Verification items for this drawing (mm, ordinates from the low corner). Coordinates: 2 decimals unless noted, no trailing zeros. Order: outer loops, then holes, each group sorted by start corner. A loop starts at its lowest first (then second) coordinate and runs counter-clockwise, first axis right, second up. Notation, with made-up numbers: (-32.5, 6) -> (-11.5, 6) arc R14 ccw to (-11.5, 14) -> close; hole circle Ø2 at (36.25, 18). An arc over 180 degrees is marked (long way). Put each result on its own line as item: value. Start each with the question number.
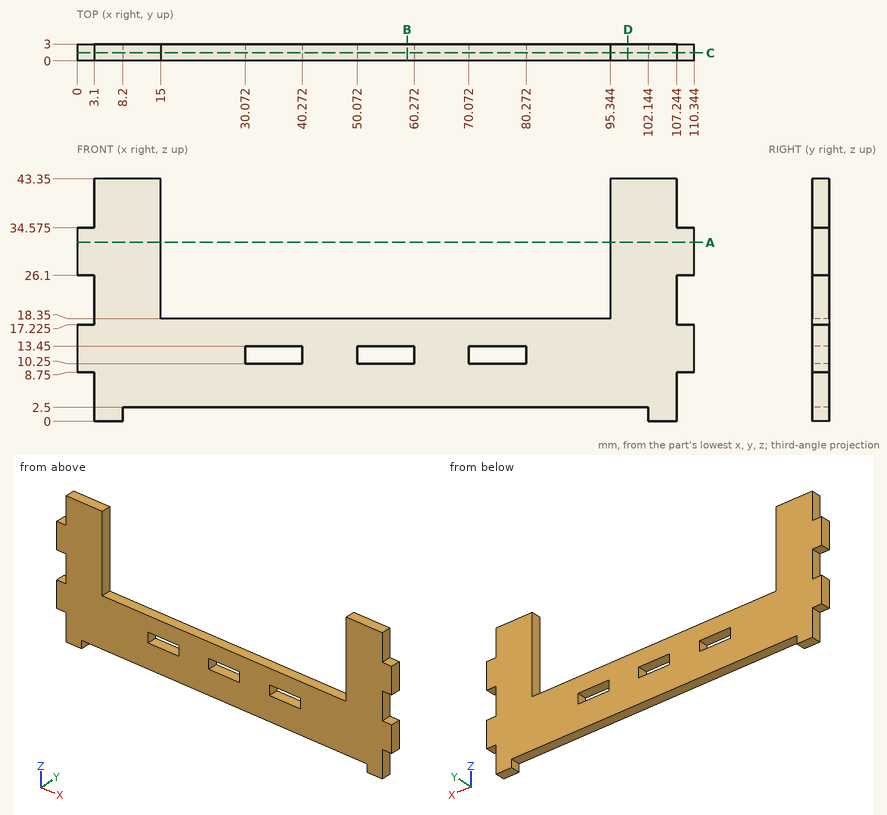
1) Sectioned sample at A-A (z = 32). Record the boundary of the cut face in (x, y) (1 decimal).
2) Sectioned sample at D-D (x = 98.5). Record the boundary of the cut face in (y, z).
3) Sectioned sample at C-C (y = 1.4). State how many separate pieces and enclosed holes the cut face has, plus the area to 3 significant figures.
4) Gauge pin test, flat ends, axial feed: pin 1 (1.5 mm diameter, centred on y = 1.5, z = 5, fed in from +X); pin 2 (0.9 mm diameter, centred on x = 1, y = 1, fed in from -Z); pin 3 (1 mm diameter, centred on x = 64.5, y = 1, fed in from -Z). Record the tip position at first contact, or that the pin passes through.
5) Scan lines: line 1 along Z through (x, y) = (55, 0.2); line 2 along X through (y, z) = (2.5, 23.5) (1 decimal); line 3 along X through (y, z) = (1.1, 32) (1 decimal). Record each from-to range of solid material in increasing order. Write a range as [from, to].
6) Sectioned sample at B-B (x = 59). Record the boundary of the cut face in (y, z).
Entries:
1. outline: (0, 0) -> (15, 0) -> (15, 3) -> (0, 3) -> close; (95.3, 0) -> (110.3, 0) -> (110.3, 3) -> (95.3, 3) -> close
2. outline: (0, 2.5) -> (3, 2.5) -> (3, 43.35) -> (0, 43.35) -> close
3. separate pieces: 1
3. enclosed holes: 3
3. area: 2,280 mm2
4. pin 1: stops at x = 107.24
4. pin 2: stops at z = 8.75
4. pin 3: stops at z = 2.5
5. line 1: z = [2.5, 10.25], [13.45, 18.35]
5. line 2: x = [3.1, 15], [95.3, 107.2]
5. line 3: x = [0, 15], [95.3, 110.3]
6. outline: (0, 2.5) -> (3, 2.5) -> (3, 10.25) -> (0, 10.25) -> close; (0, 13.45) -> (3, 13.45) -> (3, 18.35) -> (0, 18.35) -> close
